from build123d import *

# Parameters (mm, degrees)
SKETCH_1_R          = 50
EXTRUDE_1_DEPTH     = 12
FILLET_1_R          = 4
SKETCH_5_R          = 3
CUT_EXTRUDE_1_DEPTH = 3
SKETCH_7_W          = 8.05
SKETCH_7_H          = 6.15
CUT_EXTRUDE_2_DEPTH = 72.721684308


with BuildPart() as part:
    # 草图1 → 凸台-拉伸1 (new body)
    with BuildSketch(Plane(origin=(0, 0, 0), x_dir=(1, 0, 0), z_dir=(0, 1, 0))):
        with Locations(Location((0, 0, 0), (0, 0, 270))):
            Circle(SKETCH_1_R)
    extrude(amount=EXTRUDE_1_DEPTH)

    # 圆角1
    fillet_1_edges = [part.edges().sort_by_distance(p)[0] for p in [
        (0, 12, -50),
    ]]
    fillet(fillet_1_edges, radius=FILLET_1_R)

    # 草图5 → 切除-拉伸1 (cut)
    with BuildSketch(Plane(origin=(0, 12, 0), x_dir=(1, 0, 0), z_dir=(0, 1, 0))):
        with Locations(Location((-20.941763413, 21.466971597, 0), (0, 0, 270))):
            Circle(SKETCH_5_R)
        with Locations(Location((20.941763413, 21.466971597, 0), (0, 0, 90))):
            Circle(SKETCH_5_R)
        with Locations(Location((20.399845913, -22.80585614, 0), (0, 0, 270))):
            Circle(SKETCH_5_R)
        with Locations(Location((-21.471132177, -21.780666781, 0), (0, 0, 90))):
            Circle(SKETCH_5_R)
    extrude(amount=-CUT_EXTRUDE_1_DEPTH, mode=Mode.SUBTRACT)

    # 草图7 → 切除-拉伸2 (cut, through all)
    with BuildSketch(Plane(origin=(0, 12, 0), x_dir=(1, 0, 0), z_dir=(0, 1, 0))):
        Rectangle(SKETCH_7_W, SKETCH_7_H)
    extrude(amount=-CUT_EXTRUDE_2_DEPTH, mode=Mode.SUBTRACT)


solid = part.part
Here's how the part is built. I have some questions about the finished solid (model axes, mm). A direction names the side the tool comes from. Give positions to 0.01 mm unless a question says otherwise; leave off trailing zeros. Order: outer loops, then holes, each group sorted by start corner. A loop starts at its lowest first (then second) coordinate and runs counter-clockwise, first axis right, second up. Notation, with made-up numbers: (-36, -39) -> (-11, -39) arc R30 ccw to (-11, 0) -> close; hole circle Ø7 at (-31.5, 68.5). An arc over 180 degrees is marked (long way). Use a Markdown table: item, result. Add a question column.
Item 1: Will these pins go through, and if not, where does the flat tip stop? pin 1 (4 mm diameter, centred on y = 10, z = -28.5, fed in from +X); pin 2 (4 mm diameter, centred on x = 6, y = 4.5, fed in from +Z); pin 3 (5 mm diameter, centred on y = 3, z = 1, fed in from +X).
Item 2: Imagine slicing it at C-C on y = 6.5. Please give me the cut outline in (x, z) (3 decimals).
Item 3: For faces 1 (the face through (-10, 0, -1)), 2 (the face through (-22, 9, 22)), 3 (the face through (0, 6, -3.075)), which set-ups out of +Z, -Z, +X, -X, +Y, -Y let a thin tool reach every point of the face, with its end or its side?
Item 4: I need wall thicknesses on line 1 (X direction, y = 4, z = 3) (3 decimals); line 2 (Z direction, x = -40.5, y = 11); line 3 (X direction, y = 10, z = -16.5). Which ranges of each line are inside material? Lowest first, please.
Item 5: Imagine slicing it at A-A on z = 0. Please give me the cut outline in (x, y) (3 decimals).
Item 6: If we mould it in two halves opening along Z, with no side actions, what happens to faces 4 (the face through (-4.025, 6, 0)), 5 (the face through (1, 12, 10)), 6 (the face through (15.02, 3.94, 47.69))? For each: pulls with the +Z half, pulls with the -Z half, needs draft (parallel to the pull), parting line crosses it, or undercut.
Item 7: Imagine slicing it at B-B on x = 0. Please give me the cut outline in (y, z) (3 decimals), plus the area to 3 significant figures.
Data:
| question | item | result |
|---|---|---|
| 1 | pin 1 | stops at x = 42.08 |
| 1 | pin 2 | stops at z = 49.84 |
| 1 | pin 3 | stops at x = 50 |
| 2 | outline | circle Ø100 at (0, 0); hole (-4.025, -3.075) -> (4.025, -3.075) -> (4.025, 3.075) -> (-4.025, 3.075) -> close |
| 3 | face 1 | +Z, -Z, +X, -X, -Y |
| 3 | face 2 | +Y |
| 3 | face 3 | +Y, -Y |
| 4 | line 1 | x = -49.91 to -4.025, 4.025 to 49.91 |
| 4 | line 2 | z = -26.95 to 26.95 |
| 4 | line 3 | x = -46.63 to 46.63 |
| 5 | outline | (-50, 0) -> (-4.025, 0) -> (-4.025, 12) -> (-46, 12) arc R4 ccw to (-50, 8) -> close; (4.025, 0) -> (50, 0) -> (50, 8) arc R4 ccw to (46, 12) -> (4.025, 12) -> close |
| 6 | face 4 | undercut |
| 6 | face 5 | needs draft |
| 6 | face 6 | parting line crosses it |
| 7 | outline | (0, -50) -> (8, -50) arc R4 ccw to (12, -46) -> (12, -3.075) -> (0, -3.075) -> close; (0, 3.075) -> (12, 3.075) -> (12, 46) arc R4 ccw to (8, 50) -> (0, 50) -> close |
| 7 | area | 1,120 mm² |
